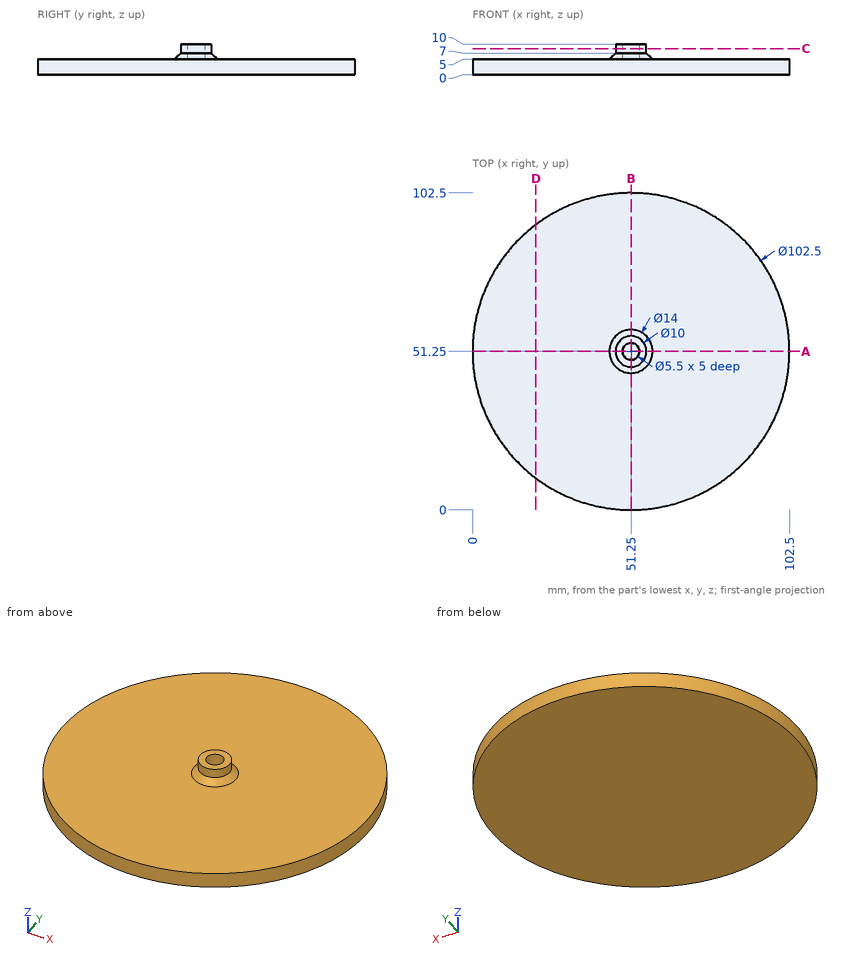
Verification items for this drawing (mm, ordinates from the low corner). Give positions to 0.01 mm unless a question says otherwise; leave off trailing zeros. Write each loop counter-clockwise with the first axis right and the second up, starting at its lowest first coordinate (ties: lowest second). Pieces come first, ordered by that corner, then holes. Notation, with made-up numbers: (-2, 25.5) - (55, 25.5) arc R22 ccw to (55, 57.5) - close; hole circle Ø6 at (-29, -39.5). An arc over 180 degrees is marked (long way). Answer as CSV lines item,"result". Start each with the question number.
1. Sectioned sample at C-C (z = 8.5). Record the boundary of the cut face in (x, y).
2. Depth check by flat-ended pin: pin 1 (1 mm diameter, centred on x = 12.5, z = 1.5, fed in from -Y); pin 2 (3 mm diameter, centred on x = 51.5, y = 50.5, fed in from +Z); pin 3 (5 mm diameter, centred on x = 28, z = 1.5, fed in from +Y). Enter the tip coordinate at first touch or a pass-through.
3. Sectioned sample at D-D (x = 20.5). Record the boundary of the cut face in (y, z).
4. Thickness scan on line 1 (Y direction, x = 51.25, z = 7.4); line 2 (Z direction, x = 76.5, y = 46); line 3 (X direction, y = 51.25, z = 6.85). Record the ranges inside material, lowest first.
5. Sectioned sample at A-A (y = 51.25). Record the boundary of the cut face in (x, z), then the cut area to 3 significant figures.
Derived:
1,outline,"circle Ø10 at (51.25, 51.25); hole circle Ø5.5 at (51.25, 51.25)"
2,pin 1,"y = 17.14"
2,pin 2,"z = 5"
2,pin 3,"y = 98.11"
3,outline,"(10.25, 0) - (92.25, 0) - (92.25, 5) - (10.25, 5) - close"
4,line 1,"46.25 to 48.5, 54 to 56.25"
4,line 2,"0 to 5"
4,line 3,"46.1 to 48.5, 54 to 56.4"
5,outline,"(0, 0) - (102.5, 0) - (102.5, 5) - (58.25, 5) - (56.25, 7) - (56.25, 10) - (54, 10) - (54, 5) - (48.5, 5) - (48.5, 10) - (46.25, 10) - (46.25, 7) - (44.25, 5) - (0, 5) - close"
5,area,"539 mm²"
